```python
from build123d import *

# Parameters (mm, degrees)
BOSS_EXTRUDE1_DEPTH      = 38.1
BOSS_EXTRUDE1_DEPTH_BACK = 38.1
SKETCH2_R                = 3.175
CUT_EXTRUDE1_DEPTH       = 12.7


with BuildPart() as part:
    # Sketch2 → Boss-Extrude1 (new, two sides: drawn at the far end of the back side and taken through both)
    with BuildSketch(Plane.XY.offset(-BOSS_EXTRUDE1_DEPTH_BACK)):
        with Locations(Location((0, 0, 0), (0, 0, 180))):
            Circle(SKETCH2_R)
    extrude(amount=BOSS_EXTRUDE1_DEPTH + BOSS_EXTRUDE1_DEPTH_BACK)

    # Sketch3 → Cut-Extrude1 (cut)
    with BuildSketch(Plane(origin=(0, 0, -38.1), x_dir=(-1, 0, 0), z_dir=(0, 0, -1))):
        with BuildLine():
            Line((1.1811, 2.947138916), (1.1811, 1.778738916))
            Line((1.1811, 1.778738916), (-1.1811, 1.778738916))
            Line((-1.1811, 1.778738916), (-1.1811, 2.947138916))
            ThreePointArc((-1.1811, 2.947138916), (0, 3.175), (1.1811, 2.947138916))
        make_face()
    extrude(amount=-CUT_EXTRUDE1_DEPTH, mode=Mode.SUBTRACT)


solid = part.part
```
Geometry: final body of the model. Coordinates: model frame, mm. A direction names the side the tool comes from. Coordinates: 2 decimals unless noted, no trailing zeros. Order: outer loops, then holes, each group sorted by start corner. A loop starts at its lowest first (then second) coordinate and runs counter-clockwise, first axis right, second up. Notation, with made-up numbers: (26.25, -8) -> (82.25, -8) arc R21 ccw to (82.25, 9) -> close; hole circle Ø3 at (10, -34). An arc over 180 degrees is marked (long way). Write each question's results on one line, items separated by ' | '. Start each with the question number.
1) First-contact query: pin 1 (3 mm diameter, centred on y = -2, z = -2.5, fed in from -X); pin 2 (0.7 mm diameter, centred on x = 0.5, y = 2.5, fed in from -Z); pin 3 (1.9 mm diameter, centred on x = 0, z = -34, fed in from +Y). Flat tips, straight axial feed; report the tip coordinate or a pass-through.
2) Cut plane D-D, the plane z = -29.5. Output: boundary loops of the cut face in (x, y) (3 decimals), and give its area (3 significant figures).
3) Cut plane B-B, the plane z = -20. Output: boundary loops of the cut face in (x, y) (3 decimals).
4) Material intervals for line 1 along X through (y, z) = (-0.25, 28); line 2 along Z through (x, y) = (-1, 2); line 3 along Y through (x, z) = (1.25, -16), sorted ascending.
5) Set-up query: faces 1 (the flat face through (0, 2, -25.4)), 2 (the flat face through (0, 0, -38.1)). Return all of +Z, -Z, +X, -X, +Y, -Y with unobstructed straight access to the full face (end or side cutting, diameter ignored); none if empty.
6) Cut plane A-A, the plane x = 0. Output: boundary loops of the cut face in (y, z) (3 decimals), and give its area (3 significant figures).
7) Cut plane C-C, the plane y = -1.25. Output: boundary loops of the cut face in (x, z).
8) Mould query, pull axis X, two halves, no side actions, for faces 3 (the cylindrical face through (0.41, -3.15, -0.53)), 4 (the flat face through (0, 0, 38.1)), 5 (the flat face through (-1.181, 2, -32)), 6 (the flat face through (1.181, 2, -32)). Classes: released by +X, released by -X, zero draft, split by the parting line, or undercut.
Checks:
1) pin 1: x = -3.14 | pin 2: z = -25.4 | pin 3: y = 1.78
2) outline: (-1.181, 1.779) -> (-1.181, 2.947) arc R3.175 ccw (long way) to (1.181, 2.947) -> (1.181, 1.779) -> close | area: 28.5 mm^2
3) outline: circle Ø6.35 at (0, 0)
4) line 1: -3.17 to 3.17 | line 2: -25.4 to 38.1 | line 3: -2.92 to 2.92
5) face 1: -Z, +Y | face 2: -Z, +X, -X, +Y, -Y
6) outline: (-3.175, -38.1) -> (1.779, -38.1) -> (1.779, -25.4) -> (3.175, -25.4) -> (3.175, 38.1) -> (-3.175, 38.1) -> close | area: 466 mm^2
7) outline: (-2.92, -38.1) -> (2.92, -38.1) -> (2.92, 38.1) -> (-2.92, 38.1) -> close
8) face 3: split by the parting line | face 4: zero draft | face 5: undercut | face 6: undercut
